Design review of the part built by this model. Coordinates are the model's own, in mm. Give positions to 0.01 mm unless a question says otherwise; leave off trailing zeros. Loops run counter-clockwise (first coordinate to the right, second up) from the corner with the lowest first, then second, coordinate; pieces in that order, holes last. Notation, with made-up numbers: (-13.5, 88.25) -> (27.5, 88.25) arc R22 cw to (27.5, 112.25) -> close; hole circle Ø6 at (89.25, -19). An arc over 180 degrees is marked (long way). Use a Markdown table: item, result. Add a question column.
1. For pin 1 Ø4.5 at (x, z) = (29, -5) entering from -Y, flat-tipped, find the tip position at first contact; note if it passes through.
2. Add section A-A (z = -3.5). State the section outline as (x, y) points, and give its area (3 significant figures).
3. Add section B-B (x = -29). State the section outline as (y, z) points, and give its area (3 significant figures).
4. Add section C-C (y = 25.5). State the section outline as (x, z) points, and give its area (3 significant figures).
5. To check wall thickness, follow line 1 (Z direction, x = -29, y = 5.5); line 2 (X direction, y = 0, z = -3.5); line 3 (X direction, y = -3.5, z = -6.25). State the ranges of each line that lie inside material, in increasing order.
```python
from build123d import *

# Parameters (mm, degrees)
SKETCH1_W           = 70
SKETCH1_H           = 60
BOSS_EXTRUDE1_DEPTH = 10
SKETCH3_R           = 2.5
CUT_EXTRUDE1_DEPTH  = 71.178344238


with BuildPart() as part:
    # Sketch1 → Boss-Extrude1 (new body)
    with BuildSketch(Plane.XY):
        Rectangle(SKETCH1_W, SKETCH1_H)
    extrude(amount=-BOSS_EXTRUDE1_DEPTH)

    # Sketch3 → Cut-Extrude1 (cut, through all)
    with BuildSketch(Plane(origin=(0, 30, 0), x_dir=(1, 0, 0), z_dir=(0, 1, 0))):
        with Locations(Location((-29, 5, 0), (0, 0, 180))):
            Circle(SKETCH3_R)
        with Locations(Location((29, 5, 0), (0, 0, 180))):
            Circle(SKETCH3_R)
    extrude(amount=-CUT_EXTRUDE1_DEPTH, mode=Mode.SUBTRACT)


solid = part.part
```
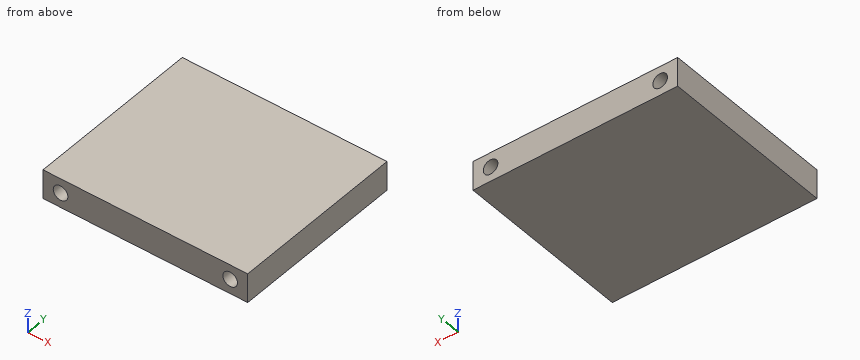
Taken from the geometry:
| question | item | result |
|---|---|---|
| 1 | pin 1 | passes through |
| 2 | outline | (-35, -30) -> (-31, -30) -> (-31, 30) -> (-35, 30) -> close; (-27, -30) -> (27, -30) -> (27, 30) -> (-27, 30) -> close; (31, -30) -> (35, -30) -> (35, 30) -> (31, 30) -> close |
| 2 | area | 3,720 mm^2 |
| 3 | outline | (-30, -10) -> (30, -10) -> (30, -7.5) -> (-30, -7.5) -> close; (-30, -2.5) -> (30, -2.5) -> (30, 0) -> (-30, 0) -> close |
| 3 | area | 300 mm^2 |
| 4 | outline | (-35, -10) -> (35, -10) -> (35, 0) -> (-35, 0) -> close; hole circle Ø5 at (-29, -5); hole circle Ø5 at (29, -5) |
| 4 | area | 661 mm^2 |
| 5 | line 1 | z = -10 to -7.5, -2.5 to 0 |
| 5 | line 2 | x = -35 to -31, -27 to 27, 31 to 35 |
| 5 | line 3 | x = -35 to -31.17, -26.83 to 26.83, 31.17 to 35 |
